from build123d import *

# Parameters (mm, degrees)
SKETCH_7_W               = 1.7
SKETCH_7_H               = 40
PATTERN_CIRCULAR_2_COUNT = 2
PATTERN_CIRCULAR_2_ANGLE = 90


with BuildPart() as part:
    # 草图6 → 旋转2 (revolve)
    with BuildSketch(Plane.XY, mode=Mode.PRIVATE) as revolve_2_sk:
        Polygon((15, 12.5), (15, 10), (-5, 10), (-5, 40), (-2.2, 40), (-1.371572875, 38), (1.371572875, 38), (2.2, 40), (5, 40), (5, 12.5), align=None)
    revolve(revolve_2_sk.sketch.rotate(Axis((-5, 0, 0), (1, 0, 0)), 90), axis=Axis((-5, 0, 0), (1, 0, 0)))

    # 草图7 → 切除-旋转3 (revolve, cut)
    with BuildSketch(Plane.XY, mode=Mode.PRIVATE) as cut_revolve_3_sk:
        with Locations((10.85, 20)):
            Rectangle(SKETCH_7_W, SKETCH_7_H)
    cut_revolve_3 = revolve(cut_revolve_3_sk.sketch.rotate(Axis((10, 40, 0), (0, -1, 0)), 180), axis=Axis((10, 40, 0), (0, -1, 0)), mode=Mode.SUBTRACT)

    # 阵列(圆周)2: 切除-旋转3 ×2 about axis
    pattern_circular_2_axis = Axis((-5, 0, 0), (-1, 0, 0))
    for i in range(1, PATTERN_CIRCULAR_2_COUNT):
        add(cut_revolve_3.rotate(pattern_circular_2_axis, i * PATTERN_CIRCULAR_2_ANGLE / (PATTERN_CIRCULAR_2_COUNT - 1)), mode=Mode.SUBTRACT)


solid = part.part
Design review of the part built by this model. Coordinates are the model's own, in mm. A direction names the side the tool comes from. Give positions to 0.01 mm unless a question says otherwise; leave off trailing zeros. Loops run counter-clockwise (first coordinate to the right, second up) from the corner with the lowest first, then second, coordinate; pieces in that order, holes last. Notation, with made-up numbers: M 9,78.25 L 51,78.25 A11 ccw 51,87.25 Z; hole C 37,42 d3. An arc over 180 degrees is marked long. Answer as a JSON object with one key per item and string values.
Item 1: We need section A-A (y = 0). State the section outline as (x, z) points.
Output values:
{"outline": "M -5,-40 L -2.2,-40 L -1.37,-38 L 1.37,-38 L 2.2,-40 L 5,-40 L 5,-12.5 L 8.3,-12.5 L 8.3,-10 L -5,-10 Z; M -5,10 L 15,10 L 15,12.5 L 5,12.5 L 5,40 L 2.2,40 L 1.37,38 L -1.37,38 L -2.2,40 L -5,40 Z; M 11.7,-12.5 L 15,-12.5 L 15,-10 L 11.7,-10 Z"}
Item 2: Wall thickness on line 1 along Y through (x, z) = (4.5, 0); line 2 along X through (y, z) = (-9, 23); line 3 along Y through (x, z) = (8, 0): over which ranges is each line inside the solid? List them lowest first.
Output values:
{"line 1": "y = -40 to -10, 10 to 40", "line 2": "x = -5 to 5", "line 3": "y = -12.5 to -10, 10 to 12.5"}
Item 3: Mouldability with a two-part tool opening along X and no side actions: class faces 1 (the face through (-5, 8, -8)), 2 (the face through (5, -9, -9)), 3 (the face through (9.2, 11.2, 1.5)) as pulls with the +X half, pulls with the -X half, needs draft (parallel to the pull), parting line crosses it, or undercut.
Output values:
{"face 1": "pulls with the -X half", "face 2": "pulls with the +X half", "face 3": "undercut"}
Item 4: Machinability: for faces 4 (the face through (0.019, 37.096, -8.238)), 5 (the face through (4.86, -3, 9.54)), 6 (the face through (10.07, -3.755, 11.923)), 7 (the face through (8.38, -0.51, -11.2)), which of the approach directions +Z, -Z, +X, -X, +Y, -Y give a long, thin tool a straight path to every point of the face, cutting with its end or side? Answer none if there is none.
Output values:
{"face 4": "none", "face 5": "+X, -X", "face 6": "+X", "face 7": "-Z"}
Item 5: We need section B-B (z = 0). State the section outline as (x, y) points, and give its area (3 significant figures).
Output values:
{"outline": "M -5,-40 L -2.2,-40 L -1.37,-38 L 1.37,-38 L 2.2,-40 L 5,-40 L 5,-12.5 L 15,-12.5 L 15,-10 L -5,-10 Z; M -5,10 L 8.3,10 L 8.3,12.5 L 5,12.5 L 5,40 L 2.2,40 L 1.37,38 L -1.37,38 L -2.2,40 L -5,40 Z; M 11.7,10 L 15,10 L 15,12.5 L 11.7,12.5 Z", "area": "627 mm2"}
Item 6: We need section C-C (x = 9.5). State the section outline as (y, z) points, and give its area (3 significant figures).
Output values:
{"outline": "M -1.62,-12.39 L -1.62,-9.87 A10 cw long 9.87,1.62 L 12.39,1.62 A12.5 ccw long Z; M 1.62,-12.39 A12.5 ccw 12.39,-1.62 L 9.87,-1.62 A10 cw 1.62,-9.87 Z", "area": "160 mm2"}
Item 7: We need section D-D (x = 3.75). State the section outline as (y, z) points, and give its area (3 significant figures).
Output values:
{"outline": "C 0,0 d80; hole C 0,0 d20", "area": "4,710 mm2"}
Item 8: For P1, Ø8, axis at x = 5, z = -6, coming from the +Y side; P2, Ø16, axis at y = 0, z = 0, coming from the +X side; P3, Ø4.5, axis at x = 10, y = 0, coming from the +Z side; P4, Ø3, axis at x = 5.5, z = 24, coming from the +Y side, all flat-tipped, find the tip position at first contact; note any pin that passes through.
Output values:
{"P1": "stops at y = 39.95", "P2": "passes through", "P3": "stops at z = 12.5", "P4": "stops at y = 33.01"}
